Autodesk Inventor part; units mm, degrees
ref_plane "YZ Plane" through (0, 0, 0) normal (1, 0, 0) x (0, 1, 0)
ref_plane "XZ Plane" through (0, 0, 0) normal (0, 1, 0) x (-1, 0, 0)
ref_plane "XY Plane" through (0, 0, 0) normal (0, 0, 1) x (1, 0, 0)
sketch "Flange Sketch" plane through (0, 0, 0) normal (0, 1, 0) x (-1, 0, 0)
  circle A0 centre (0, 0) radius 114.3
  circle A1 centre (0, 0) radius 58.039
  circle A2 centre (0, 0) radius 95.25 construction
  line L0 (0, 0) -> (-36.4506, -87.9995) construction
  line L1 (0, 0) -> (0, -95.25) construction
  dimension "outerDiam" = 228.6
  dimension "innerDiam" = 116.078
  dimension "boltCircle" = 190.5
  dimension "boltOffsetAngle" = 22.5
extrude "Flange Extrusion" add sketch "Flange Sketch" along normal blind 15.875
hole "Bolt Hole" at (36.4506, 0, -87.9995) direction (0, 1, 0) diameter 19.05 depth 15.875
pattern_circular "Bolt Hole Pattern" count 8 over 360 about axis through (0, -10, 0) along (0, 1, 0) of "Bolt Hole"
equation "\"nominalSize\" = 101.6"
properties part number "AWWA-C207-B4-S"
The model under review builds one solid part; all positions refer to its coordinate system, in mm. Round coordinates to 2 decimals unless told otherwise and drop trailing zeros. Loops run counter-clockwise (first coordinate to the right, second up) from the corner with the lowest first, then second, coordinate; pieces in that order, holes last. Notation, with made-up numbers: (1, 30.25) -> (19, 30.25) arc R33 cw to (19, 69.25) -> close; hole circle Ø2 at (-34, -35). An arc over 180 degrees is marked (long way). Return JSON: item names as keys, results as strings.
(1) Add section C-C on x = 92. Write out the cut boundary in (y, z) (3 decimals), plus the area to 3 significant figures.
Solved:
{"outline": "(0, -67.827) -> (15.875, -67.827) -> (15.875, -45.095) -> (0, -45.095) -> close; (0, -27.806) -> (15.875, -27.806) -> (15.875, 27.806) -> (0, 27.806) -> close; (0, 45.095) -> (15.875, 45.095) -> (15.875, 67.827) -> (0, 67.827) -> close", "area": "1,600 mm2"}
(2) Add section D-D on y = 7. State how many separate pieces and enclosed holes the cut face has, plus the area to 3 significant figures.
Solved:
{"separate pieces": "1", "enclosed holes": "9", "area": "28,200 mm2"}
(3) Add section B-B on z = 0. Write out the cut boundary in (x, y) (3 decimals).
Solved:
{"outline": "(-114.3, 0) -> (-58.039, 0) -> (-58.039, 15.875) -> (-114.3, 15.875) -> close; (58.039, 0) -> (114.3, 0) -> (114.3, 15.875) -> (58.039, 15.875) -> close"}
(4) Add section A-A on x = 0. Write out the cut boundary in (y, z) (3 decimals).
Solved:
{"outline": "(0, -114.3) -> (15.875, -114.3) -> (15.875, -58.039) -> (0, -58.039) -> close; (0, 58.039) -> (15.875, 58.039) -> (15.875, 114.3) -> (0, 114.3) -> close"}
(5) For pin 1 (1.5 mm diameter, centred on x = 44.5, y = 7.5, fed in from -Z); pin 2 (6 mm diameter, centred on x = 43.5, y = 12.5, fed in from +Z); pin 3 (5 mm diameter, centred on y = 8.5, z = -90.5, fed in from -X), all flat-tipped, find the tip position at first contact; note any pin that passes through.
Solved:
{"pin 1": "z = -105.6", "pin 2": "z = 106.88", "pin 3": "x = -72.94"}
(6) For line 1 (Z direction, x = -87, y = 2.5); line 2 (Z direction, x = 84, y = 7); line 3 (Z direction, x = 0, y = 10.25), list the stretches that pass through material, from the lowest coordinate up.
Solved:
{"line 1": "-74.13 to -45.92, -26.98 to 26.98, 45.92 to 74.13", "line 2": "-77.51 to -45.1, -27.81 to 27.81, 45.1 to 77.51", "line 3": "-114.3 to -58.04, 58.04 to 114.3"}
(7) The part is to be moulded in two halves that separate along Z. For faces 1 (the cylindrical face through (114.19, 7.83, -5.03)), 2 (the cylindrical face through (-40.09, 8.05, -96.8)), 3 (the cylindrical face through (40.09, 8.05, 96.8)), 4 (the flat face through (52, 0, 27)), say which applies: released by +Z, released by -Z, zero draft, split by the parting line, or undercut.
Solved:
{"face 1": "split by the parting line", "face 2": "undercut", "face 3": "undercut", "face 4": "zero draft"}
